Design review of the part built by this model. Coordinates are the model's own, in mm. Coordinates: 2 decimals unless noted, no trailing zeros. Write each loop counter-clockwise with the first axis right and the second up, starting at its lowest first coordinate (ties: lowest second). Pieces come first, ordered by that corner, then holes. Notation, with made-up numbers: (45, 2.5) - (60, 2.5) arc R30 ccw to (60, 25.5) - close; hole circle Ø4 at (61.5, 63.5). An arc over 180 degrees is marked (long way). Use a Markdown table: item, result.
Autodesk Inventor part; units mm, degrees
ref_plane "YZ Plane" through (0, 0, 0) normal (1, 0, 0) x (0, 1, 0)
ref_plane "XZ Plane" through (0, 0, 0) normal (0, 1, 0) x (-1, 0, 0)
ref_plane "XY Plane" through (0, 0, 0) normal (0, 0, 1) x (1, 0, 0)
sketch "Sketch1" plane through (0, 0, 0) normal (0, 0, 1) x (1, 0, 0)
  line L0 (-28.59, -15) -> (28.59, -15)
  line L1 (28.59, -15) -> (28.59, 15)
  line L2 (28.59, 15) -> (-28.59, 15)
  line L3 (-28.59, 15) -> (-28.59, -15)
  line L4 (-28.59, -15) -> (28.59, 15) construction
  line L5 (28.59, -15) -> (-28.59, 15) construction
  point P0 (0, 0)
  dimension "d0" = 57.18
  dimension "d1" = 30
extrude "Plate1" add sketch "Sketch1" along normal blind 1.5
sketch "Sketch2" plane through (-27.09, -15, 0) normal (-1, 0, 0) x (0, -1, 0)
  line L0 (-30, 0) -> (0, 0)
  line L1 (0, 0) -> (0, 33)
  line L2 (0, 33) -> (-30, 33)
  line L3 (-30, 33) -> (-30, 0)
edge flange "Flange1" height 33 angle 90 thickness 1.5 bend radius 0.31 thickness toward (-1, 0, 0) relief tear relief width 1.5 relief depth 0.75 corner gap 0.31 corner form 0 edges at (-28.59, 0, 1.5) (28.59, 0, 1.5) wall of the first edge with corners at (-27.09, 15, 0) (-27.09, -15, 0) (-27.09, -15, 33) (-27.09, 15, 33)
bend "Bend1"
corner "Corner1"
sketch "Sketch3" plane through (28.59, -15, 33) normal (1, 0, 0) x (0, 0, -1)
  circle A0 centre (17, 15) radius 9.96
  line L0 (0, 30) -> (31.19, 30)
  line L1 (31.19, 0) -> (0, 0)
  line L2 (31.19, 30) -> (13.9636, 24.4859)
  line L3 (31.19, 0) -> (13.9636, 5.5141)
  line L4 (0, 30) -> (0, 0)
  point P0 (33, 15)
  dimension "d13" = 19.92
  dimension "d14" = 0
  dimension "d15" = 16
extrude "Cut1" cut sketch "Sketch3" against normal blind 57.18 contours A0 L3 L1 L4 L0 L2
sketch "Sketch17" plane through (28.59, -15, 1.81) normal (1, 0, 0) x (0, 0, -1)
  circle A0 centre (-21.19, 15) radius 0.7835
  circle A1 centre (-14.19, 22) radius 0.7835
  circle A2 centre (-7.19, 15) radius 0.7835
  circle A3 centre (-14.19, 8) radius 0.7835
  point P0 (1.81, 15)
hole "Hole7" at (28.59, 0, 23) at (28.59, 7, 16) at (28.59, 0, 9) at (28.59, -7, 16) direction (-1, 0, 0) diameter 2.1 depth 1.5
sketch "Sketch18" plane through (-28.59, -15, 1.81) normal (-1, 0, 0) x (0, 0, 1)
  circle A0 centre (14.19, 22) radius 0.7835
  circle A1 centre (21.19, 15) radius 0.7835
  circle A2 centre (14.19, 8) radius 0.7835
  circle A3 centre (7.19, 15) radius 0.7835
  point P0 (-1.81, 15)
hole "Hole8" at (-28.59, 7, 16) at (-28.59, 0, 23) at (-28.59, -7, 16) at (-28.59, 0, 9) direction (1, 0, 0) diameter 2.1 depth 1.5
sketch "Sketch19" plane through (0, 0, 1.5) normal (0, 0, 1) x (1, 0, 0)
  point P0 (0, 0)
sketch "Sketch21" plane through (-28.59, -15, 1.81) normal (-1, 0, 0) x (0, 0, 1)
  point P0 (-1.81, 15)
sketch "Sketch22" plane through (-28.59, -15, 1.81) normal (-1, 0, 0) x (0, 0, 1)
  circle A0 centre (14.19, 15) radius 1.75
  point P0 (-1.81, 15)
sketch "Sketch23" plane through (-28.59, -15, 1.81) normal (-1, 0, 0) x (0, 0, 1)
  point P0 (-1.81, 15)
hole "Hole10" at (-28.59, 0, 16) direction (1, 0, 0) diameter 7.2 depth 1.5
sketch "Sketch24" plane through (28.59, -15, 1.81) normal (1, 0, 0) x (0, 0, -1)
  circle A0 centre (-14.19, 15) radius 1.2295
  point P0 (1.81, 15)
hole "Hole11" at (28.59, 0, 16) direction (-1, 0, 0) diameter 5.2 depth 1.5
sketch "Sketch25" plane through (0, 0, 1.5) normal (0, 0, 1) x (1, 0, 0)
  circle A0 centre (7.525, 7.5) radius 0.7835
  circle A1 centre (7.525, -12.5) radius 0.7835
  circle A2 centre (-7.525, -12.5) radius 0.7835
  circle A3 centre (-7.525, 7.5) radius 0.7835
  point P0 (0, 0)
hole "Hole12" at (7.525, 7.5, 1.5) at (7.525, -12.5, 1.5) at (-7.525, 7.5, 1.5) at (-7.525, -12.5, 1.5) direction (0, 0, -1) diameter 2.1 depth 1.5
equation "\"d90\" = Thickness"
equation "\"d97\" = Thickness"
equation "\"d111\" = Thickness"
equation "\"d118\" = Thickness"
equation "\"d125\" = Thickness"
equation "\"d2\" = Thickness"
equation "\"d3\" = BendReliefWidth"
equation "\"d4\" = BendReliefDepth"
equation "\"d5\" = MinimumRemnant"
equation "\"d6\" = TransitionRadius"
equation "\"d9\" = BendRadius"
equation "\"d10\" = CornerReliefSize"
equation "\"d11\" = GapSize"
equation "\"d12\" = JacobiRadiusSize"
equation "\"BendReliefWidth\" = Thickness"
equation "\"BendReliefDepth\" = 0.5 * Thickness"
equation "\"CornerReliefSize\" = 4 * Thickness"
equation "\"MinimumRemnant\" = 2 * Thickness"
equation "\"TransitionRadius\" = BendRadius"
equation "\"JacobiRadiusSize\" = BendRadius"
equation "\"GapSize\" = Thickness"
properties part number "axis_20_bottom_frame" material "Aluminum 6061-AHC"
(1) For pin 1 (1.7 mm diameter, centred on y = 0, z = 23, fed in from +X); pin 2 (2.5 mm diameter, centred on x = -7.525, y = 7.5, fed in from +Z), all flat-tipped, find the tip position at first contact; note any pin that passes through.
Determined:
| item | result |
|---|---|
| pin 1 | through |
| pin 2 | z = 1.5 |
(2) Take a section at A-A on y = -12.5. Write out the cut boundary in (x, z) (3 decimals).
Determined:
| item | result |
|---|---|
| outline | (-28.59, 1.81) arc R1.81 ccw to (-26.78, 0) - (-8.575, 0) - (-8.575, 1.5) - (-26.78, 1.5) arc R0.31 cw to (-27.09, 1.81) - (-27.09, 9.62) - (-28.59, 9.62) - close; (-6.475, 0) - (6.475, 0) - (6.475, 1.5) - (-6.475, 1.5) - close; (8.575, 0) - (26.78, 0) arc R1.81 ccw to (28.59, 1.81) - (28.59, 9.62) - (27.09, 9.62) - (27.09, 1.81) arc R0.31 cw to (26.78, 1.5) - (8.575, 1.5) - close |
(3) Take a section at C-C on y = 0. State how many separate pieces and enclosed holes the cut face has, and give its area (3 significant figures).
Determined:
| item | result |
|---|---|
| separate pieces | 7 |
| enclosed holes | 0 |
| area | 127 mm2 |
(4) For L1, parallel to X at y = -7, z = 20.75; L2, parallel to Y at x = -27.65, z = 16; L3, parallel to Z at x = -27.65, y = 0, list the stretches that pass through material, from the lowest coordinate up. Write a range as from..to.
Determined:
| item | result |
|---|---|
| L1 | -28.59..-27.09, 27.09..28.59 |
| L2 | -10.46..-8.05, -5.95..-3.6, 3.6..5.95, 8.05..10.46 |
| L3 | 0.22..7.95, 10.05..12.4, 19.6..21.95, 24.05..25.96 |
(5) Draft analysis for pull direction X (two halves, no side actions). For faces 1 (the cylindrical face through (28.07, 0.21, 0.54)), 2 (the cylindrical face through (-7.84, -13.5, 0.74)), 3 (the cylindrical face through (-27.83, -0.158, 12.403)), state which applies: +X half, -X half, draft (parallel to the pull), parting line (faces both ways), or undercut.
Determined:
| item | result |
|---|---|
| face 1 | +X half |
| face 2 | undercut |
| face 3 | draft |
(6) Take a section at B-B on z = 3.5. Write out the cut boundary in (x, y).
Determined:
| item | result |
|---|---|
| outline | (-28.59, -14.46) - (-27.09, -14.46) - (-27.09, 14.46) - (-28.59, 14.46) - close; (27.09, -14.46) - (28.59, -14.46) - (28.59, 14.46) - (27.09, 14.46) - close |
